Autodesk Inventor part; units mm, degrees
ref_plane "YZ Plane" through (0, 0, 0) normal (1, 0, 0) x (0, 1, 0)
ref_plane "XZ Plane" through (0, 0, 0) normal (0, 1, 0) x (-1, 0, 0)
ref_plane "XY Plane" through (0, 0, 0) normal (0, 0, 1) x (1, 0, 0)
sketch "Sketch1" plane through (0, 0, 0) normal (0, 0, 1) x (1, 0, 0)
  line L0 (-9.6332, 12.3072) -> (10.3668, 12.3072)
  line L1 (10.3668, 12.3072) -> (10.3668, -12.6928)
  line L2 (10.3668, -12.6928) -> (-9.6332, -12.6928)
  line L3 (-9.6332, -12.6928) -> (-9.6332, 12.3072)
  line L4 (-4.3832, -2.6928) -> (5.1168, -2.6928)
  line L5 (5.1168, -2.6928) -> (5.1168, -7.7928)
  line L6 (5.1168, -7.7928) -> (-4.3832, -7.7928)
  line L7 (-4.3832, -7.7928) -> (-4.3832, -2.6928)
  line L8 (-1.0332, -2.6928) -> (-1.0332, -7.7928)
  line L9 (1.7668, -2.6928) -> (1.7668, -7.7928)
  line L10 (-1.0332, -2.6928) -> (-1.0332, 0.3072)
  line L11 (1.7668, -2.6928) -> (1.7668, 0.3072)
  line L12 (-1.0332, 0.3072) -> (-6.6332, 12.3072)
  line L13 (1.7668, 0.3072) -> (7.3668, 12.3072)
  line L14 (-1.0332, -7.7928) -> (-1.0332, -12.6928)
  line L15 (1.7668, -7.7928) -> (1.7668, -12.6928)
  point P0 (0, 0)
  dimension "d0" = 20
  dimension "d1" = 25
  dimension "d2" = 3.35
  dimension "d3" = 3.35
  dimension "d4" = 2.8
  dimension "d5" = 5.1
  dimension "d6" = 5.25
  dimension "d7" = 9.5
  dimension "d9" = 15
  dimension "d10" = 4.9
  dimension "d11" = 3
  dimension "d12" = 3
  dimension "d13" = 3
  dimension "d14" = 3
extrude "Extrusion1" add sketch "Sketch1" along normal blind 3 contours L0 L12 L10 L4 L7 L6 L14 L2 L3 | L0 L1 L2 L15 L6 L5 L4 L11 L13
extrude "Extrusion2" add sketch "Sketch1" against normal blind 5
chamfer "Chamfer1" distance 12 distance2 3 1 edges at (0.3668, 12.3072, 0) measured on face at (-0.0999, 8.3072, 0)
sketch "Sketch3" plane through (0, 0, 3) normal (0, 0, 1) x (1, 0, 0)
  line L0 (-9.6332, 12.3072) -> (-9.6332, -12.6928)
  line L1 (-9.6332, -12.6928) -> (-1.0332, -12.6928)
  line L2 (-1.0332, -12.6928) -> (-1.0332, -7.7928)
  line L3 (-1.0332, -7.7928) -> (-4.3832, -7.7928)
  line L4 (-4.3832, -7.7928) -> (-4.3832, -2.6928)
  line L5 (-4.3832, -2.6928) -> (-1.0332, -2.6928)
  line L6 (-1.0332, -2.6928) -> (-1.0332, 0.3072)
  line L7 (-1.0332, 0.3072) -> (-6.6332, 12.3072)
  line L8 (-6.6332, 12.3072) -> (-9.6332, 12.3072)
  line L9 (10.3668, -12.6928) -> (10.3668, 12.3072)
  line L10 (10.3668, 12.3072) -> (7.3668, 12.3072)
  line L11 (7.3668, 12.3072) -> (1.7668, 0.3072)
  line L12 (1.7668, 0.3072) -> (1.7668, -2.6928)
  line L13 (1.7668, -2.6928) -> (5.1168, -2.6928)
  line L14 (5.1168, -2.6928) -> (5.1168, -7.7928)
  line L15 (5.1168, -7.7928) -> (1.7668, -7.7928)
  line L16 (1.7668, -7.7928) -> (1.7668, -12.6928)
  line L17 (1.7668, -12.6928) -> (10.3668, -12.6928)
  point P0 (0, 0)
  point P1 (-6.6332, 5.8072)
  point P2 (7.3668, 5.8072)
  point P3 (-6.6332, -9.6928)
  point P4 (7.3668, -9.6928)
  dimension "d24" = 25
  dimension "d25" = 6.5
  dimension "d26" = 3
  dimension "d27" = 4.9
  dimension "d28" = 3
  dimension "d29" = 3
  dimension "d37" = 5.25
  dimension "d38" = 3
  dimension "d39" = 3
hole "Hole1" at (-6.6332, 5.8072, 3) at (7.3668, 5.8072, 3) at (-6.6332, -9.6928, 3) at (7.3668, -9.6928, 3) direction (0, 0, -1) diameter 2.5 end through all
fillet "Fillet1" radius 1.5 2 edges at (-6.6332, 12.3072, 0) (7.3668, 12.3072, 0)
fillet "Fillet2" radius 2 4 edges at (-9.6332, 12.3072, -1) (10.3668, 12.3072, -1) (10.3668, -12.6928, -1) (-9.6332, -12.6928, -1)
sketch "Sketch4" plane through (0, 0, 3) normal (0, 0, 1) x (1, 0, 0)
  line L0 (-13.7185, 14.5378) -> (16.1134, 14.5378)
  line L1 (16.1134, 14.5378) -> (16.1134, -15.8403)
  line L2 (16.1134, -15.8403) -> (-13.7185, -15.8403)
  line L3 (-13.7185, -15.8403) -> (-13.7185, 14.5378)
  point P0 (0, 0)
extrude "Extrusion4" cut sketch "Sketch4" against normal blind 3
equation "\"d3\" = d2"
equation "\"d6\" = -0.5 * d7 + 0.5 * d0"
equation "\"d12\" = d11"
equation "\"d14\" = d13"
properties part number "3DP_PLA_Part_Detector_Top_Half" material "ABS Plastic"
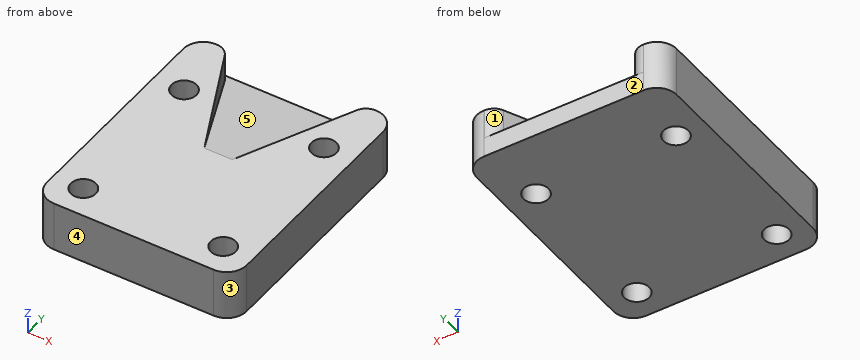
The listing builds one solid part. Answer for the finished solid, in the listing's coordinates (mm). Face numbers are marked on the shaded views. A direction names the side the tool comes from. Coordinates: 2 decimals unless noted, no trailing zeros. Loops run counter-clockwise (first coordinate to the right, second up) from the corner with the lowest first, then second, coordinate; pieces in that order, holes last.
1) Find section B-B on y = 6.5. Write down the section's boundary in (x, z).
2) A flat-ended cylindrical pin translates along its axis: pin 1 Ø2 at (x, y) = (-6.63, 5.81) entering from +Z. Find the tip coordinate at first contact, or state that the pin passes through.
3) Find section D-D on z = -4.55. Write down the section's boundary in (x, y), then the cut area to 3 significant figures.
4) Determine the mould class of the marked faces 3, 4 and 5 for opening direction X: pulls with the +X half, pulls with the -X half, needs draft (parallel to the pull), parting line crosses it, or undercut.
5) A tool of negligible diameter and unlimited length cuts with its end or side. For the marked faces 1 and 2, from which of +Z, -Z, +X, -X, +Y, -Y can it reach the whole face along a straight path? Write none if from no direction.
6) Find section A-A on z = -2.05. Write down the section's boundary in (x, y).
7) Find the intervals of material crossed by L1, parallel to X at y = 6.5, z = -3.8; L2, parallel to Y at x = 6.75, z = -3.8; L3, parallel to X at y = 9, z = -0.3, in increasing order.
8) Find section C-C on x = 0.5. Write down the section's boundary in (y, z), then the cut area to 3 significant figures.
Values:
1. outline: (-9.63, -5) - (-7.67, -5) - (-7.67, 0) - (-9.63, 0) - close; (-5.59, -5) - (6.33, -5) - (6.33, 0) - (4.66, 0) - (4.66, -1.55) - (-3.92, -1.55) - (-3.92, 0) - (-5.59, 0) - close; (8.41, -5) - (10.37, -5) - (10.37, 0) - (8.41, 0) - close
2. pin 1: passes through
3. outline: (-9.63, -10.69) arc R2 ccw to (-7.63, -12.69) - (8.37, -12.69) arc R2 ccw to (10.37, -10.69) - (10.37, 10.31) arc R2 ccw to (8.37, 12.31) - (-7.63, 12.31) arc R2 ccw to (-9.63, 10.31) - close; hole circle Ø2.5 at (-6.63, -9.69); hole circle Ø2.5 at (-6.63, 5.81); hole circle Ø2.5 at (7.37, -9.69); hole circle Ø2.5 at (7.37, 5.81)
3. area: 477 mm2
4. face 3: pulls with the +X half
4. face 4: needs draft
4. face 5: undercut
5. face 1: +Z, +Y
5. face 2: +Z, -Z, +X, -X, +Y
6. outline: (-9.63, -10.69) arc R2 ccw to (-7.63, -12.69) - (8.37, -12.69) arc R2 ccw to (10.37, -10.69) - (10.37, 10.31) arc R2 ccw to (8.37, 12.31) - (8.32, 12.31) arc R1.5 ccw to (6.96, 11.44) - (5.59, 8.51) - (-4.86, 8.51) - (-6.23, 11.44) arc R1.5 ccw to (-7.59, 12.31) - (-7.63, 12.31) arc R2 ccw to (-9.63, 10.31) - close; hole circle Ø2.5 at (-6.63, -9.69); hole circle Ø2.5 at (-6.63, 5.81); hole circle Ø2.5 at (7.37, -9.69); hole circle Ø2.5 at (7.37, 5.81)
7. L1: x = -9.63 to -7.67, -5.59 to 6.33, 8.41 to 10.37
7. L2: y = -12.69 to -10.78, -8.61 to 4.72, 6.89 to 12.31
7. L3: x = -9.63 to -5.09, 5.82 to 10.37
8. outline: (-12.69, -5) - (12.31, -5) - (12.31, -3) - (0.31, 0) - (-12.69, 0) - close
8. area: 107 mm2
